Autodesk Inventor part; units mm, degrees
ref_plane "YZ Plane" through (0, 0, 0) normal (1, 0, 0) x (0, 1, 0)
ref_plane "XZ Plane" through (0, 0, 0) normal (0, 1, 0) x (-1, 0, 0)
ref_plane "XY Plane" through (0, 0, 0) normal (0, 0, 1) x (1, 0, 0)
sketch "Sketch1" plane through (0, 0, 0) normal (0, 0, 1) x (1, 0, 0)
  line L0 (0, 0) -> (9.525, 0)
  line L1 (9.525, 0) -> (9.525, 25.4)
  line L2 (9.525, 25.4) -> (0, 25.4)
  line L3 (0, 25.4) -> (0, 0)
  line L4 (0, 0) -> (38.1, 0)
  line L5 (38.1, 0) -> (38.1, 6.35)
  line L6 (38.1, 6.35) -> (0, 6.35)
  line L7 (0, 6.35) -> (0, 0)
  line L8 (9.525, 25.4) -> (12.7508, 25.4)
  line L9 (12.7508, 25.4) -> (12.7508, 0) construction
  line L10 (12.7508, 0) -> (9.525, 0)
  line L11 (9.525, 0) -> (9.525, 25.4)
  point P0 (9.525, 6.35)
  dimension "d0" = 9.525
  dimension "d1" = 25.4
  dimension "d2" = 38.1
  dimension "d3" = 6.35
  dimension "d4" = 3.2258
extrude "Extrusion1" add sketch "Sketch1" along normal blind 76.2
sketch "Sketch2" plane through (9.525, 0, 0) normal (0, 1, 0) x (1, 0, 0)
  line L0 (28.575, -76.2) -> (0, -76.2)
  line L1 (14.2875, -76.2) -> (14.2875, 0) construction
  line L2 (28.575, 0) -> (0, 0)
  line L3 (28.575, 0) -> (28.575, -76.2)
  point P0 (-9.525, 0)
  point P1 (21.4312, -63.5)
  point P2 (21.4312, -38.1)
  point P3 (21.4312, -12.7)
  point P4 (7.1437, -63.5)
  point P5 (7.1437, -38.1)
  point P6 (7.1437, -12.7)
  dimension "d8" = 7.1437
  dimension "d9" = 14.2875
  dimension "d10" = 12.7
  dimension "d13" = 25.4
  dimension "d16" = 14.2875
hole "Hole1" at (30.9563, 0, 63.5) at (30.9563, 0, 38.1) at (30.9563, 0, 12.7) at (16.6688, 0, 63.5) at (16.6688, 0, 38.1) at (16.6688, 0, 12.7) direction (0, 1, 0) diameter 3.81 end through all countersink diameter 7.0866 countersink angle 82
fillet "Fillet1" radius 3.175 5 edges at (9.525, 15.875, 76.2) (9.525, 15.875, 0) (38.1, 3.175, 76.2) (38.1, 3.175, 0) (0, 0, 38.1)
fillet "Fillet2" radius 3.175 1 edges at (0, 25.4, 38.1)
properties part number "Arena Top Bracket"
For this review, take the finished solid that the model builds, in its own axes (mm). A direction names the side the tool comes from. Coordinates: 2 decimals unless noted, no trailing zeros. Write each loop counter-clockwise with the first axis right and the second up, starting at its lowest first coordinate (ties: lowest second). Pieces come first, ordered by that corner, then holes. Notation, with made-up numbers: (73.25, 44) - (87.25, 44) arc R24 cw to (87.25, 83) - close; hole circle Ø10 at (12, -14). An arc over 180 degrees is marked (long way). Answer in a Markdown table with one row per item. Add a question column.
Q1. Tool access review of faces 1 (the flat face through (9.525, 16, 38)), 2 (the conical face through (29.18, 1.77, 37.17)), 3 (the cylindrical face through (8.57, 16.008, 75.295)): name each direction out of +Z, -Z, +X, -X, +Y, -Y from which nothing blocks a thin tool from reaching the whole face with its end or side.
Q2. Draft analysis for pull direction Z (two halves, no side actions). For faces 4 (the cylindrical face through (8.62, 16.008, 0.955)), 5 (the conical face through (29, 1.77, 13.14)), 6 (the flat face through (20.4, 0, 37.6)), state which applies: +Z half, -Z half, draft (parallel to the pull), parting line (faces both ways), or undercut.
Q3. We need section A-A, the plane z = 12.7. Count the separate pieces of the cut face and the enclosed holes in it, and give its area (3 significant figures).
Q4. We need section D-D, the plane x = 25.5. State the section outline as (y, z) points, and give its area (3 significant figures).
Q5. We need section C-C, the plane y = 10. State the section outline as (x, z) points (3 decimals), and give its area (3 significant figures).
Q6. For probe 1 along X at (y, z) = (4.45, 63.5); probe 2 along X at (y, z) = (2, 39); probe 3 along Z at (x, y) = (30.5, 1.25), list the stretches that pass through material, from the lowest coordinate up.
Q7. We need section B-B, the plane y = 4.5. State the section outline as (x, z) points (3 decimals).
Q8. For P1, Ø12, axis at x = 23, z = 15, coming from the +Y side; P2, Ø5, axis at x = 16.67, z = 38.1, coming from the -Y side, all flat-tipped, find the tip position at first contact; note any pin that passes through.
Answer list:
| question | item | result |
|---|---|---|
| 1 | face 1 | +Z, -Z, +X, +Y |
| 1 | face 2 | -Y |
| 1 | face 3 | +Z, +X, +Y |
| 2 | face 4 | -Z half |
| 2 | face 5 | undercut |
| 2 | face 6 | draft |
| 3 | separate pieces | 3 |
| 3 | enclosed holes | 0 |
| 3 | area | 364 mm2 |
| 4 | outline | (0, 0) - (6.35, 0) - (6.35, 76.2) - (0, 76.2) - close |
| 4 | area | 484 mm2 |
| 5 | outline | (0, 0) - (6.35, 0) arc R3.175 ccw to (9.525, 3.175) - (9.525, 73.025) arc R3.175 ccw to (6.35, 76.2) - (0, 76.2) - close |
| 5 | area | 721 mm2 |
| 6 | probe 1 | x = 0 to 14.76, 18.57 to 29.05, 32.86 to 38.1 |
| 6 | probe 2 | x = 0.23 to 14.99, 18.35 to 29.28, 32.64 to 38.1 |
| 6 | probe 3 | z = 0 to 10.29, 15.11 to 35.69, 40.51 to 61.09, 65.91 to 76.2 |
| 7 | outline | (0, 0) - (34.925, 0) arc R3.175 ccw to (38.1, 3.175) - (38.1, 73.025) arc R3.175 ccw to (34.925, 76.2) - (0, 76.2) - close; hole circle Ø3.81 at (16.669, 12.7); hole circle Ø3.81 at (16.669, 38.1); hole circle Ø3.81 at (16.669, 63.5); hole circle Ø3.81 at (30.956, 12.7); hole circle Ø3.81 at (30.956, 38.1); hole circle Ø3.81 at (30.956, 63.5) |
| 8 | P1 | stops at y = 6.35 |
| 8 | P2 | stops at y = 1.2 |
